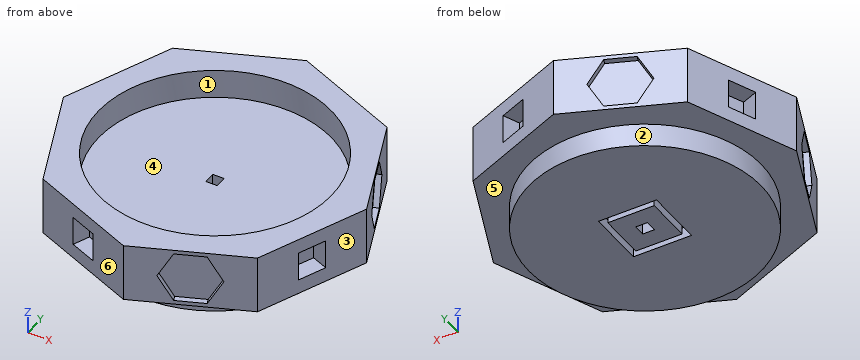
```python
from build123d import *

# Parameters (mm, degrees)
F1_DEPTH  = 50
F2_W      = 25
F2_H      = 25
F3_DEPTH  = 15
F4_W      = 25
F4_H      = 25
F5_DEPTH  = 15
F6_W      = 25
F6_H      = 25
F7_DEPTH  = 15
F8_W      = 25
F8_H      = 25
F9_DEPTH  = 15
F11_DEPTH = 5
F13_DEPTH = 5
F15_DEPTH = 5
F17_DEPTH = 5
F18_R     = 100
F19_DEPTH = 25
F20_R     = 100
F21_DEPTH = 20
F23_W     = 50
F23_H     = 50
F24_DEPTH = 10
F25_W     = 40
F25_H     = 40
F26_DEPTH = 10
F27_W     = 10
F27_H     = 10
F28_DEPTH = 45


with BuildPart() as f1:
    # F0 (on Top) → F1 (new body)
    with BuildSketch(Plane.XY):
        Polygon((-92.3879532511, -92.3879532511), (0, -130.6562964876), (92.3879532511, -92.3879532511), (130.6562964876, 0), (92.3879532511, 92.3879532511), (0, 130.6562964876), (-92.3879532511, 92.3879532511), (-130.6562964876, 0), align=None)
    extrude(amount=F1_DEPTH)

    # F2 (on face) → F3 (cut)
    with BuildSketch(Plane(origin=(-46.1939766256, -111.5221248694, 0), x_dir=(0.9238795325, -0.3826834324, 0), z_dir=(-0.3826834324, -0.9238795325, 0))):
        with Locations((0, 25)):
            Rectangle(F2_W, F2_H)
    extrude(amount=-F3_DEPTH, mode=Mode.SUBTRACT)

    # F4 (on face) → F5 (cut)
    with BuildSketch(Plane(origin=(-111.5221248694, 46.1939766256, 0), x_dir=(-0.3826834324, -0.9238795325, 0), z_dir=(-0.9238795325, 0.3826834324, 0))):
        with Locations((0, 25)):
            Rectangle(F4_W, F4_H)
    extrude(amount=-F5_DEPTH, mode=Mode.SUBTRACT)

    # F6 (on face) → F7 (cut)
    with BuildSketch(Plane(origin=(46.1939766256, 111.5221248694, 0), x_dir=(-0.9238795325, 0.3826834324, 0), z_dir=(0.3826834324, 0.9238795325, 0))):
        with Locations((0, 25)):
            Rectangle(F6_W, F6_H)
    extrude(amount=-F7_DEPTH, mode=Mode.SUBTRACT)

    # F8 (on face) → F9 (cut)
    with BuildSketch(Plane(origin=(111.5221248694, -46.1939766256, 0), x_dir=(0.3826834324, 0.9238795325, 0), z_dir=(0.9238795325, -0.3826834324, 0))):
        with Locations((0, 25)):
            Rectangle(F8_W, F8_H)
    extrude(amount=-F9_DEPTH, mode=Mode.SUBTRACT)

    # F10 (on face) → F11 (cut)
    with BuildSketch(Plane(origin=(46.1939766256, -111.5221248694, 0), x_dir=(0.9238795325, 0.3826834324, 0), z_dir=(0.3826834324, -0.9238795325, 0))):
        Polygon((12.4999989995, 3.3493643278), (25, 24.9999988448), (12.5000010005, 46.650634517), (-12.4999989995, 46.6506356722), (-25, 25.0000011552), (-12.5000010005, 3.349365483), align=None)
    extrude(amount=-F11_DEPTH, mode=Mode.SUBTRACT)

    # F12 (on face) → F13 (cut)
    with BuildSketch(Plane(origin=(111.5221248694, 46.1939766256, 0), x_dir=(-0.3826834324, 0.9238795325, 0), z_dir=(0.9238795325, 0.3826834324, 0))):
        Polygon((12.4999987427, 3.3493641795), (25, 24.9999985481), (12.5000012573, 46.6506343687), (-12.4999987427, 46.6506358205), (-25, 25.0000014519), (-12.5000012573, 3.3493656313), align=None)
    extrude(amount=-F13_DEPTH, mode=Mode.SUBTRACT)

    # F14 (on face) → F15 (cut)
    with BuildSketch(Plane(origin=(-111.5221248694, -46.1939766256, 0), x_dir=(0.3826834324, -0.9238795325, 0), z_dir=(-0.9238795325, -0.3826834324, 0))):
        Polygon((12.5, 46.6506350946), (-12.5, 46.6506350946), (-25, 25), (-12.5, 3.3493649054), (12.5, 3.3493649054), (25, 25), align=None)
    extrude(amount=-F15_DEPTH, mode=Mode.SUBTRACT)

    # F16 (on face) → F17 (cut)
    with BuildSketch(Plane(origin=(-46.1939766256, 111.5221248694, 0), x_dir=(-0.9238795325, -0.3826834324, 0), z_dir=(-0.3826834324, 0.9238795325, 0))):
        Polygon((12.5, 46.6506350946), (-12.5, 46.6506350946), (-25, 25), (-12.5, 3.3493649054), (12.5, 3.3493649054), (25, 25), align=None)
    extrude(amount=-F17_DEPTH, mode=Mode.SUBTRACT)

    # F18 (on face) → F19 (cut)
    with BuildSketch(Plane.XY.offset(50)):
        Circle(F18_R)
    extrude(amount=-F19_DEPTH, mode=Mode.SUBTRACT)

    # F20 (on face) → F21 (join)
    with BuildSketch(Plane(origin=(0, 0, 0), x_dir=(1, 0, 0), z_dir=(0, 0, -1))):
        Circle(F20_R)
    extrude(amount=F21_DEPTH)


with BuildPart() as f1_1:
    # F22: moved
    add(f1.part.moved(Location((0, 0, 10))))

    # F23 (on face) → F24 (cut)
    with BuildSketch(Plane(origin=(0, 0, -10), x_dir=(1, 0, 0), z_dir=(0, 0, -1))):
        Rectangle(F23_W, F23_H)
    extrude(amount=-F24_DEPTH, mode=Mode.SUBTRACT)

    # F25 (on face) → F26 (join)
    with BuildSketch(Plane(origin=(0, 0, 0), x_dir=(1, 0, 0), z_dir=(0, 0, -1))):
        Rectangle(F25_W, F25_H)
    extrude(amount=F26_DEPTH)

    # F27 (on face) → F28 (cut)
    with BuildSketch(Plane(origin=(0, 0, -10), x_dir=(1, 0, 0), z_dir=(0, 0, -1))):
        Rectangle(F27_W, F27_H)
    extrude(amount=-F28_DEPTH, mode=Mode.SUBTRACT)


solid = f1_1.part
```
Source: CAD feature listing. Evaluate the final solid. Frame: model axes, mm. Face numbers are marked on the shaded views. A direction names the side the tool comes from. Coordinates: 2 decimals unless noted, no trailing zeros. Write each loop counter-clockwise with the first axis right and the second up, starting at its lowest first coordinate (ties: lowest second). Pieces come first, ordered by that corner, then holes. Notation, with made-up numbers: M 88,26 L 136,26 A13 ccw 136,33 Z; hole C 73.25,18 d11. An arc over 180 degrees is marked long. Answer as a JSON object with one key per item and string values.
1. Contact query for flat-ended pins moving along their axis: P1, Ø11.5, axis at x = -50.5, y = -100.5, coming from the -Z side; P2, Ø10, axis at y = 30.5, z = 40.5, coming from the +X side; P3, Ø12, axis at x = 37.5, z = 44, coming from the +Y side. Output: stop coordinate, or through.
Evaluation:
{"P1": "z = 10", "P2": "x = 120.09", "P3": "y = 117.61"}
2. Cut plane B-B on x = 74. Output: boundary loops of the cut face in (y, z), plus the area to 3 significant figures.
Evaluation:
{"outline": "M -100,10 L -67.26,10 L -67.26,-10 L 67.26,-10 L 67.26,10 L 100,10 L 100,60 L 67.26,60 L 67.26,35 L -67.26,35 L -67.26,60 L -100,60 Z", "area": "9,330 mm^2"}
3. Draft query along Y for the marked faces 4, 5 and 6. Return one class per face: released by +Y, released by -Y, zero draft, split by the parting line, or undercut.
Evaluation:
{"face 4": "undercut", "face 5": "zero draft", "face 6": "released by -Y"}
4. Cut plane D-D on x = -46. Output: boundary loops of the cut face in (y, z).
Evaluation:
{"outline": "M -111.6,10 L -88.79,10 L -88.79,-10 L 88.79,-10 L 88.79,10 L 111.6,10 L 111.6,13.35 L 106.19,13.35 L 106.19,56.65 L 111.6,56.65 L 111.6,60 L 88.79,60 L 88.79,35 L -88.79,35 L -88.79,60 L -111.6,60 L -111.6,47.5 L -95.37,47.5 L -95.37,22.5 L -111.6,22.5 Z"}
5. Ray query, L1, parallel to Y at x = 0, z = 49.5; L2, parallel to Z at x = -61.5, y = -102; L3, parallel to Y at x = 44, z = 49. Return the intervals inside material, ascending.
Evaluation:
{"L1": "-130.66 to -100, 100 to 130.66", "L2": "10 to 60", "L3": "-107.02 to -89.8, 89.8 to 112.43"}
6. Access query for the marked faces 1, 2 and 3. Directions: +Z, -Z, +X, -X, +Y, -Y. A direction counts if a zero-diameter tool reaches every point of the face in a straight line with its end or side. Return the directions, or none.
Evaluation:
{"face 1": "+Z", "face 2": "-Z", "face 3": "+Z, -Z, +X, -Y"}
7. Cut plane A-A on z = 5. Output: boundary loops of the cut face in (x, y).
Evaluation:
{"outline": "C 0,0 d200; hole M -5,-5 L 5,-5 L 5,5 L -5,5 Z"}
8. Cut plane C-C on y = -84.5. Output: boundary loops of the cut face in (x, z), plus the area to 3 significant figures.
Evaluation:
{"outline": "M -95.66,10 L -53.48,10 L -53.48,-10 L 53.48,-10 L 53.48,10 L 95.66,10 L 95.66,60 L 53.48,60 L 53.48,35 L -53.48,35 L -53.48,60 L -95.66,60 Z", "area": "9,030 mm^2"}
